Work out the finished part from the listing and answer in its coordinate system (mm). A direction names the side the tool comes from. Coordinates: 2 decimals unless noted, no trailing zeros. Order: outer loops, then holes, each group sorted by start corner. A loop starts at its lowest first (then second) coordinate and runs counter-clockwise, first axis right, second up.
1. The part is cut by section B-B, the plane y = 2. Give the vertices of the cut face in (x, z), then the cut area to 3 significant figures.
2. Determine the mould class of faces 3 (the flat face through (-17.1, 0.4, 16.6)), 4 (the flat face through (0, 0, 63.5)), 5 (the flat face through (0.4, 17.1, 16.6)) for opening direction Y: +Y half, -Y half, draft (parallel to the pull), parting line (faces both ways), or undercut.
3. The part is cut by section C-C, the plane z = 39. Give the vertices of the cut face in (x, y).
4. Find the intervals of material crossed by probe 1 along Y at (x, z) = (1.5, 68); probe 2 along Z at (x, y) = (6, 22); probe 3 along Z at (x, y) = (-3.5, 1), in increasing order.
5. Flat-ended cylindrical pins translate along their axes: pin 1 Ø1.5 at (y, z) = (4, 29.5) entering from -X (3 decimals); pin 2 Ø1 at (x, y) = (-7.5, -1.5) entering from +Z; pin 3 Ø2 at (y, z) = (-10, 9) entering from +X. Find the tip coordinate at first contact, or state that the pin passes through.
6. A tool of negligible diameter and unlimited length cuts with its end or side. For faces 1 (the flat face through (-1, 0, 0)), 2 (the cylindrical face through (5.866, -2.432, 48.022)), from which of +Z, -Z, +X, -X, +Y, -Y can it reach the whole face along a straight path? Write none if from no direction.
7. The part is cut by section A-A, the plane x = 0. Give the vertices of the cut face in (y, z) (3 decimals).
8. The part is cut by section D-D, the plane x = -5.5. Give the vertices of the cut face in (y, z).
```python
from build123d import *

# Parameters (mm, degrees)
F0_W          = 50.8
F0_H          = 50.8
F4_R          = 6.35
F5_DEPTH      = 25.4
F5_DEPTH_BACK = 12.7


with BuildPart() as f3:
    # F0 (on Top) → F3 section 0
    with BuildSketch(Plane.XY, mode=Mode.PRIVATE) as f3_s0:
        Rectangle(F0_W, F0_H)
    loft([f3_s0.sketch, Vertex(0, 0, 50.8)])

    # F4 (on offset) → F5 (join, two sides)
    with BuildSketch(Plane.XY.offset(50.8)) as f5_sk:
        Circle(F4_R)
    extrude(amount=-F5_DEPTH)
    extrude(f5_sk.sketch, amount=F5_DEPTH_BACK)

    # F6 (on face) → F7 (revolve)
    with BuildSketch(Plane.XY.offset(63.5)):
        with BuildLine():
            Line((0, -6.35), (0, -8.255))
            ThreePointArc((0, -8.255), (8.255, 0), (0, 8.255))
            Line((0, 8.255), (0, 6.35))
            ThreePointArc((0, 6.35), (4.4901280605, 4.4901280605), (6.35, 0))
            ThreePointArc((6.35, 0), (4.4901280605, -4.4901280605), (0, -6.35))
        make_face()
    revolve(axis=Axis((0, 0, 63.5), (0, -1, 0)))


solid = f3.part
```
Geometry says:
1. outline: (-25.4, 0) - (25.4, 0) - (6.03, 38.75) - (6.03, 58.23) arc R8.01 ccw (long way) to (-6.03, 58.23) - (-6.03, 38.75) - close; hole (-6.03, 63.5) - (6.03, 63.5) arc R6.03 ccw to start
1. area: 1,570 mm2
2. face 3: draft
2. face 4: undercut
2. face 5: +Y half
3. outline: (-5.9, -5.9) - (-2.35, -5.9) arc R6.35 ccw to (2.35, -5.9) - (5.9, -5.9) - (5.9, -2.35) arc R6.35 ccw to (5.9, 2.35) - (5.9, 5.9) - (2.35, 5.9) arc R6.35 ccw to (-2.35, 5.9) - (-5.9, 5.9) - (-5.9, 2.35) arc R6.35 ccw to (-5.9, -2.35) - close
4. probe 1: y = -6.76 to -4.22, 4.22 to 6.76
4. probe 2: z = 0 to 6.8
4. probe 3: z = 0 to 63.5, 68.7 to 70.91
5. pin 1: stops at x = -11.025
5. pin 2: stops at z = 67.63
5. pin 3: stops at x = 21.4
6. face 1: -Z, +X, -X, +Y, -Y
6. face 2: none
7. outline: (-25.4, 0) - (25.4, 0) - (6.35, 38.1) - (6.35, 58.225) arc R8.255 ccw (long way) to (-6.35, 58.225) - (-6.35, 38.1) - close; hole (-6.35, 63.5) - (6.35, 63.5) arc R6.35 ccw to start
8. outline: (-25.4, 0) - (25.4, 0) - (5.5, 39.8) - (3.17, 39.8) - (3.17, 58.23) arc R6.16 ccw (long way) to (-3.17, 58.23) - (-3.17, 39.8) - (-5.5, 39.8) - close; hole (-3.17, 63.5) - (3.17, 63.5) arc R3.17 ccw to start
